Build history of the part. All positions in model axes, mm. Face numbers are marked on the shaded views. A direction names the side the tool comes from. Coordinates: 2 decimals unless noted, no trailing zeros. Loops run counter-clockwise (first coordinate to the right, second up) from the corner with the lowest first, then second, coordinate; pieces in that order, holes last. Notation, with made-up numbers: (-15.5, 58) -> (25.5, 58) arc R32 ccw to (25.5, 90) -> close; hole circle Ø5 at (56, 61). An arc over 180 degrees is marked (long way). One line per item, written item: value. Start each with the question number.
Autodesk Inventor part; units mm, degrees
ref_plane "YZ Plane" through (0, 0, 0) normal (1, 0, 0) x (0, 1, 0)
ref_plane "XZ Plane" through (0, 0, 0) normal (0, 1, 0) x (-1, 0, 0)
ref_plane "XY Plane" through (0, 0, 0) normal (0, 0, 1) x (1, 0, 0)
sketch "Boceto1" plane through (0, 0, 0) normal (0, 1, 0) x (-1, 0, 0)
  circle A0 centre (0, 0) radius 14
  circle A1 centre (0, 14) radius 2.1
  circle A2 centre (0, 0) radius 11
  line L0 (0, 18.1) -> (19, 18.1)
  arc A3 (0, 18.1) -> (-18.1, 0) centre (0, 0) ccw
  line L1 (0, 0) -> (5.461, 0)
  arc A4 (0, 11.4) -> (-11.4, 0) centre (0, 0) ccw
  line L2 (0, 11.4) -> (19, 11.4)
  circle A5 centre (0, -14) radius 2.1
  line L3 (0, -18.1) -> (19, -18.1)
  arc A6 (-18.1, 0) -> (0, -18.1) centre (0, 0) ccw
  arc A7 (-11.4, 0) -> (0, -11.4) centre (0, 0) ccw
  line L4 (0, -11.4) -> (19, -11.4)
  circle A8 centre (-14, 0) radius 2.1
  circle A9 centre (0, 0) radius 19
  line L5 (19, 11.4) -> (19, 18.1)
  line L6 (19, -11.4) -> (19, -18.1)
  point P0 (8.1265, 11.4)
  point P1 (8.1265, 18.1)
  point P2 (8.1265, -11.4)
  point P3 (8.1265, -18.1)
  dimension "d0" = 28
  dimension "d1" = 4.2
  dimension "d3" = 22
  dimension "d12" = 11.4
  dimension "d18" = 4.2
  dimension "d19" = 38
extrude "Extrusión1" add sketch "Boceto1" along normal blind 8 contours L2 A4 A7 L4 A0 A5 A8 A1 | A0 A1 A8 A5 L4 A9 L3 A6 A3 L0 L2 | A9 L0 L5 L2 | L4 L6 L3 A9
sketch "Boceto2" plane through (0, 0, 0) normal (0, -1, 0) x (1, 0, 0)
  arc A0 (0, -18.5) -> (0, 18.5) centre (0, 0) ccw
  line L0 (0, 18.5) -> (-19, 18.5)
  line L1 (0, 22.5) -> (-19, 22.5)
  line L2 (0, -18.5) -> (-19, -18.5)
  line L3 (0, -22.5) -> (-19, -22.5)
  arc A1 (0, -22.5) -> (0, 22.5) centre (0, 0) ccw
  line L4 (-19, 18.1) -> (0, 18.1)
  line L5 (-19, 18.1) -> (-19, 18.5)
  line L6 (-19, -18.1) -> (-19, -11.4)
  line L7 (-19, -18.1) -> (-19, -18.5)
  line L8 (-19, 22.5) -> (-19, 24.19)
  line L9 (-19, 18.5) -> (-19, 22.5)
  line L10 (-19, -18.5) -> (-19, -22.5)
  line L11 (-19, -22.5) -> (-19, -24.4563)
  point P0 (-8.1265, 18.5)
  point P1 (-8.1265, 18.1)
  point P2 (-8.1265, 22.5)
  point P3 (-8.1265, -18.5)
  point P4 (-8.1265, -22.5)
  dimension "d14" = 37
extrude "Extrusión2" add sketch "Boceto2" along normal blind 35
sketch "Boceto3" plane through (0, 0, 0) normal (0, 1, 0) x (1, 0, 0)
  line L0 (0, 18.1) -> (-19, 18.1)
  line L1 (-8.1265, 18.1) -> (0, 18.1)
  line L2 (-8.1265, -11.4) -> (-8.1265, -18.1)
  arc A0 (0, -18.1) -> (0, 18.1) centre (0, 0) ccw
  line L3 (-8.1265, -18.1) -> (0, -18.1)
  arc A1 (-8.1265, -16.1731) -> (0, 18.1) centre (0, 0) ccw
  line L4 (-8.1265, -22.5) -> (-8.1265, -18.5)
  line L5 (-8.1265, -18.1) -> (-8.1265, -22.5)
  line L6 (-8.1265, -22.5) -> (0, -22.5)
  line L7 (-19, 22.5) -> (0, 22.5)
  line L8 (-8.1265, 22.5) -> (0, 22.5)
  arc A2 (0, -22.5) -> (0, 22.5) centre (0, 0) ccw
  line L9 (-19, -22.5) -> (-19, 22.5)
  line L10 (-8.1265, 18.1) -> (-19, 18.1)
  line L11 (-19, 22.5) -> (-8.1265, 22.5)
  line L12 (0, -22.5) -> (-19, -22.5)
  line L13 (-8.1265, -22.5) -> (-19, -22.5)
  line L14 (-19, -11.4) -> (-19, -18.1)
  line L15 (-19, -22.5) -> (-19, -18.1)
  line L16 (-19, -18.1) -> (-8.1265, -18.1)
  line L17 (-19, -18.1) -> (0, -18.1)
extrude "Extrusión3" add sketch "Boceto3" along normal blind 8 contours L0 L9 L7 A2 L6 L4 L5 L3 A0 | L5 L4 L12 L9 L16
sketch "Boceto4" plane through (0, -35, 0) normal (0, -1, 0) x (1, 0, 0)
  line L0 (0, 19.5) -> (-19, 19.5)
  line L1 (-19, 22.5) -> (-19, 18.5)
  line L2 (-19, 22.5) -> (-19, 19.5)
  line L3 (0, -19.5) -> (-19, -19.5)
  line L4 (-19, -22.5) -> (-19, -11.4)
  line L5 (-19, -22.5) -> (-19, -19.5)
  line L6 (-19, -22.5) -> (0, -22.5)
  line L7 (-19, -22.5) -> (0, -22.5)
  arc A0 (0, -22.5) -> (0, 22.5) centre (0, 0) ccw
  line L8 (-19, 22.5) -> (0, 22.5)
  line L9 (0, 22.5) -> (-19, 22.5)
  arc A1 (0, -19.5) -> (0, 19.5) centre (0, 0) ccw
  arc A2 (0, -22.5) -> (0, 22.5) centre (0, 0) ccw
extrude "Extrusión4" add sketch "Boceto4" along normal blind 70
sketch "Boceto5" plane through (0, -105, 0) normal (0, -1, 0) x (1, 0, 0)
  line L0 (0, -22.5) -> (-19, -22.5)
  line L1 (0, -22.5) -> (-19, -22.5)
  line L2 (-19, -22.5) -> (-19, -11.4)
  line L3 (-19, 22.5) -> (0, 22.5)
  line L4 (-19, -22.5) -> (-19, 22.5)
  arc A0 (0, -22.5) -> (0, 22.5) centre (0, 0) ccw
extrude "Extrusión5" add sketch "Boceto5" along normal blind 3
sketch "Boceto6" plane through (-19, 0, 11.4) normal (-1, 0, 0) x (0, 0, 1)
  line L0 (-33.9, 8) -> (-48.9, 8)
  line L1 (-48.9, 8) -> (-48.9, -32)
  line L2 (-48.9, -108) -> (-33.9, -108)
  line L3 (-33.9, -108) -> (-33.9, 8)
  circle A0 centre (-41.4, -53) radius 2.6
  line L4 (-48.9, -32) -> (-48.9, -108)
  line L5 (-48.9, -12) -> (-33.9, -12)
  circle A1 centre (-41.4, -12) radius 2.6
  line L6 (-11.4, 2) -> (-11.4, -20.5205)
  line L7 (-48.9, -50) -> (-33.9, -50)
  line L8 (-33.9, 8) -> (-33.9, -108)
  circle A2 centre (-41.4, -88) radius 2.6
  line L9 (11.1, 8) -> (26.1, 8)
  line L10 (26.1, 8) -> (26.1, -32)
  line L11 (26.1, -108) -> (11.1, -108)
  line L12 (11.1, -108) -> (11.1, 8)
  circle A3 centre (18.6, -53) radius 2.6
  line L13 (26.1, -32) -> (26.1, -108)
  line L14 (26.1, -12) -> (11.1, -12)
  circle A4 centre (18.6, -12) radius 2.6
  line L15 (26.1, -50) -> (11.1, -50)
  line L16 (11.1, 8) -> (11.1, -108)
  circle A5 centre (18.6, -88) radius 2.6
  point P0 (-11.4, 0)
  point P1 (11.1, 8)
  dimension "d25" = 15
  dimension "d26" = 5.2
  dimension "d27" = 5.2
  dimension "d28" = 20
extrude "Extrusión6" add sketch "Boceto6" against normal blind 10 contours L3 L5 A1 L1 L0 | L3 L7 L4 L1 L5 A1 | L3 L2 L4 L7 | L9 L10 L14 A4 L12 | L14 A4 L10 L13 L15 L12 | L15 L13 L11 L12
properties part number "motor-fastening"
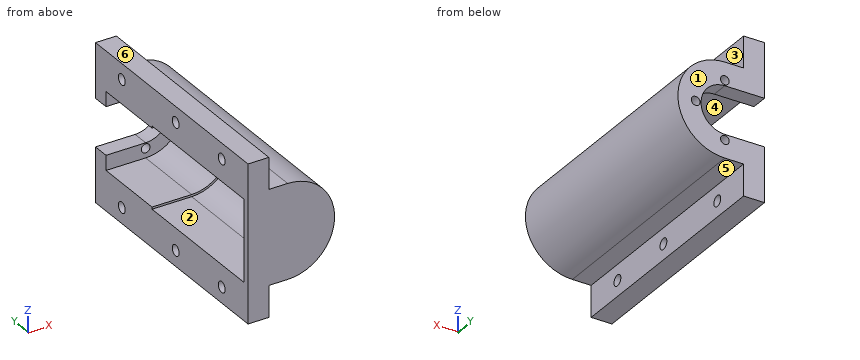
Item 1: Tool access for the marked faces 4, 5 and 6: list every direction of +Z, -Z, +X, -X, +Y, -Y with a clear straight run to the whole face (end or side of a thin tool).
Item 2: Band-saw the part on A-A, the plane z = -30. List the corners of the cut face in (x, y).
Item 3: Band-saw the part on B-B, the plane y = -12. List the corners of the cut face in (x, z), and give its area (3 significant figures).
Item 4: Two-plate mould, pull along Y, no slides. Class the marked faces 1, 2 and 3: +Y half, -Y half, draft (parallel to the pull), parting line (faces both ways), or undercut.
Item 5: Probe probe 1 along Z at (x, y) = (0, 2); probe 2 along Y at (x, z) = (-13, -30); probe 3 along Z at (x, y) = (-14, -12). List the from-to ranges inside material, lowest first.
Item 6: Band-saw the part on C-C, the plane y = -39.5. List the corners of the cut face in (x, z).
Item 7: Drop flat-ended pins along their axis: pin 1 Ø2 at (x, y) = (14.5, -39) entering from +Z; pin 2 Ø1 at (x, y) = (17.5, -85.5) entering from +Z; pin 3 Ø6.5 at (x, z) = (0, 14) entering from +Y; pin 4 Ø8.5 at (y, z) = (-88, -30) entering from +X. Give the stop position or say it passes through.
Item 8: Band-saw the part on D-D, the plane z = 14. List the corners of the cut face in (x, y).
Worked out:
1. face 4: -X
1. face 5: -Z, +X, +Y, -Y
1. face 6: +Z, +X, -X, +Y, -Y
2. outline: (-19, -108) -> (-9, -108) -> (-9, -90.6) -> (-19, -90.6) -> close; (-19, -85.4) -> (-9, -85.4) -> (-9, -55.6) -> (-19, -55.6) -> close; (-19, -50.4) -> (-9, -50.4) -> (-9, -14.6) -> (-19, -14.6) -> close; (-19, -9.4) -> (-9, -9.4) -> (-9, 8) -> (-19, 8) -> close
3. outline: (-19, -37.5) -> (-9, -37.5) -> (-9, -32.6) -> (-19, -32.6) -> close; (-19, -27.4) -> (-9, -27.4) -> (-9, -22.5) -> (0, -22.5) arc R22.5 ccw to (0, 22.5) -> (-9, 22.5) -> (-9, 27.4) -> (-19, 27.4) -> (-19, 18.5) -> (0, 18.5) arc R18.5 cw to (0, -18.5) -> (-19, -18.5) -> close; (-19, 32.6) -> (-9, 32.6) -> (-9, 37.5) -> (-19, 37.5) -> close
3. area: 606 mm²
4. face 1: +Y half
4. face 2: undercut
4. face 3: draft
5. probe 1: z = -22.5 to -16.1, -11.9 to -11.4, 11.4 to 11.9, 16.1 to 22.5
5. probe 2: y = -108 to -90.6, -85.4 to -55.6, -50.4 to -14.6, -9.4 to 8
5. probe 3: z = -37.5 to -32.6, -27.4 to -18.5, 18.5 to 27.4, 32.6 to 37.5
6. outline: (-19, -37.5) -> (-9, -37.5) -> (-9, -22.5) -> (0, -22.5) arc R22.5 ccw to (0, 22.5) -> (-9, 22.5) -> (-9, 37.5) -> (-19, 37.5) -> (-19, 19.5) -> (0, 19.5) arc R19.5 cw to (0, -19.5) -> (-19, -19.5) -> close
7. pin 1: stops at z = 18
7. pin 2: stops at z = 14.74
7. pin 3: stops at y = 8
7. pin 4: stops at x = -9
8. outline: (-19, -108) -> (17.61, -108) -> (17.61, 8) -> (2.1, 8) -> (2.1, 0) -> (12.09, 0) -> (12.09, -35) -> (13.57, -35) -> (13.57, -105) -> (-19, -105) -> close; (-19, 0) -> (-2.1, 0) -> (-2.1, 8) -> (-19, 8) -> close
